CAD build for the part. Positions are in the model's coordinates, mm. A direction names the side the tool comes from. Round coordinates to 2 decimals unless told otherwise and drop trailing zeros. Loops run counter-clockwise (first coordinate to the right, second up) from the corner with the lowest first, then second, coordinate; pieces in that order, holes last. Notation, with made-up numbers: M -27,-12 L 15,-12 A30 cw 15,12 Z; hole C 14.25,40 d4. An arc over 180 degrees is marked long. Use a Markdown table: item, result. Add a question column.
(1) Which spindle directions (+Z, -Z, +X, -X, +Y, -Y) get a long thin tool onto all of the face, cutting with end or side? Do faces 1 (the face through (57, 0, 173)), 2 (the face through (57, -35, 225.474)), 3 (the face through (69.434, -24, 12)), 4 (the face through (22, 35.86, 148)), 5 (the face through (57, -35, 122.143)). Say none if no direction does.
(2) Band-saw the part on C-C, the plane z = 183. Write the cut outline in (x, y).
(3) Band-saw the part on A-A, the plane x = 47.5. Write the cut outline in (y, z).
(4) Flat gauge pins, fed straight in: P1, Ø12.5, axis at x = 55, z = 196.5, coming from the -Y side; P2, Ø7.5, axis at x = 60.5, z = 177.5, coming from the +Y side; P3, Ø20, axis at x = 60.5, y = -26, coming from the +Z side. Where does each tip first touch, or does it go through?
(5) Band-saw the part on D-D, the plane x = 6. Write the cut outline in (y, z).
(6) Wall check: L1, parallel to Z at x = 65.5, y = -51.5; L2, parallel to Y at x = 5, z = 234.5; L3, parallel to Y at x = 47, z = 135. Give the ranges that are in metal, low to high.
(7) Band-saw the part on B-B, the plane y = -36. Write the cut outline in (x, z).
(8) Two-plate mould, pull along Z, no slides. Class faces 6 (the face through (57, -69.594, 173)), 7 (the face through (34, -24, 0)), 8 (the face through (22, -41, 275)), 9 (the face through (50, -3, 25)): released by +Z, released by -Z, zero draft, split by the parting line, or undercut.
from build123d import *

# Parameters (mm, degrees)
F0_W     = 69.4335103035
F0_H     = 70.5661773682
F1_DEPTH = 25
F2_W     = 44.6875952184
F2_H     = 35.8601175249
F3_DEPTH = 250
F4_DEPTH = 121
F5_W     = 69.5940330625
F5_H     = 103.3312529325
F7_DEPTH = 25


# Not quite as in the source:
# - the program builds the solid bodies; features that only make, move or delete a surface that nothing else refers to are left out


with BuildPart() as f1:
    # F0 (on Top) → F1 (new body)
    with BuildSketch(Plane.XY):
        with Locations((34.7167551517, 35.2830886841)):
            Rectangle(F0_W, F0_H)
    extrude(amount=F1_DEPTH)

    # F2 (on face) → F3 (join)
    with BuildSketch(Plane.XY.offset(25)):
        with Locations((22.3437976092, 17.9300587624)):
            Rectangle(F2_W, F2_H)
    extrude(amount=F3_DEPTH)

    # F4 (add): a face of the model
    f4_faces = [f1.faces().sort_by_distance(p)[0] for p in [
        (24.0077180628, 0, 131.5089430654),
    ]]
    extrude(f4_faces, amount=F4_DEPTH)

    # F5 (on face) → F7 (join)
    with BuildSketch(Plane.YZ.offset(44.6875952184)):
        with Locations((-34.7970165312, 173.8082841039)):
            Rectangle(F5_W, F5_H)
    extrude(amount=F7_DEPTH)


solid = f1.part
Return value:
| question | item | result |
|---|---|---|
| 1 | face 1 | +Z, +X, +Y |
| 1 | face 2 | +Z, +X, +Y, -Y |
| 1 | face 3 | -Z, +X, +Y, -Y |
| 1 | face 4 | +Z, +X, -X, +Y |
| 1 | face 5 | +X, +Y, -Y |
| 2 | outline | M 0,-121 L 44.69,-121 L 44.69,-69.59 L 69.69,-69.59 L 69.69,0 L 44.69,0 L 44.69,35.86 L 0,35.86 Z |
| 3 | outline | M -121,0 L 70.57,0 L 70.57,25 L -121,25 Z; M -69.59,122.14 L 0,122.14 L 0,225.47 L -69.59,225.47 Z |
| 4 | P1 | y = -69.59 |
| 4 | P2 | y = 0 |
| 4 | P3 | z = 225.47 |
| 5 | outline | M -121,0 L 70.57,0 L 70.57,25 L 35.86,25 L 35.86,275 L -121,275 Z |
| 6 | L1 | 0 to 25, 122.14 to 225.47 |
| 6 | L2 | -121 to 35.86 |
| 6 | L3 | -69.59 to 0 |
| 7 | outline | M 0,0 L 69.43,0 L 69.43,25 L 44.69,25 L 44.69,122.14 L 69.69,122.14 L 69.69,225.47 L 44.69,225.47 L 44.69,275 L 0,275 Z |
| 8 | face 6 | zero draft |
| 8 | face 7 | released by -Z |
| 8 | face 8 | released by +Z |
| 8 | face 9 | undercut |
